Here's the drawing with two shaded views (mm, measured from the low corner). I have some questions. Give positions to 0.01 mm unless a question says otherwise; leave off trailing zeros. Write each loop counter-clockwise with the first axis right and the second up, starting at its lowest first coordinate (ties: lowest second). Pieces come first, ordered by that corner, then holes. Notation, with made-up numbers: (31.25, -9) - (38.25, -9) arc R4 cw to (38.25, -3) - close; hole circle Ø2 at (24.5, 18). An arc over 180 degrees is marked (long way). Write item = value, one per line.
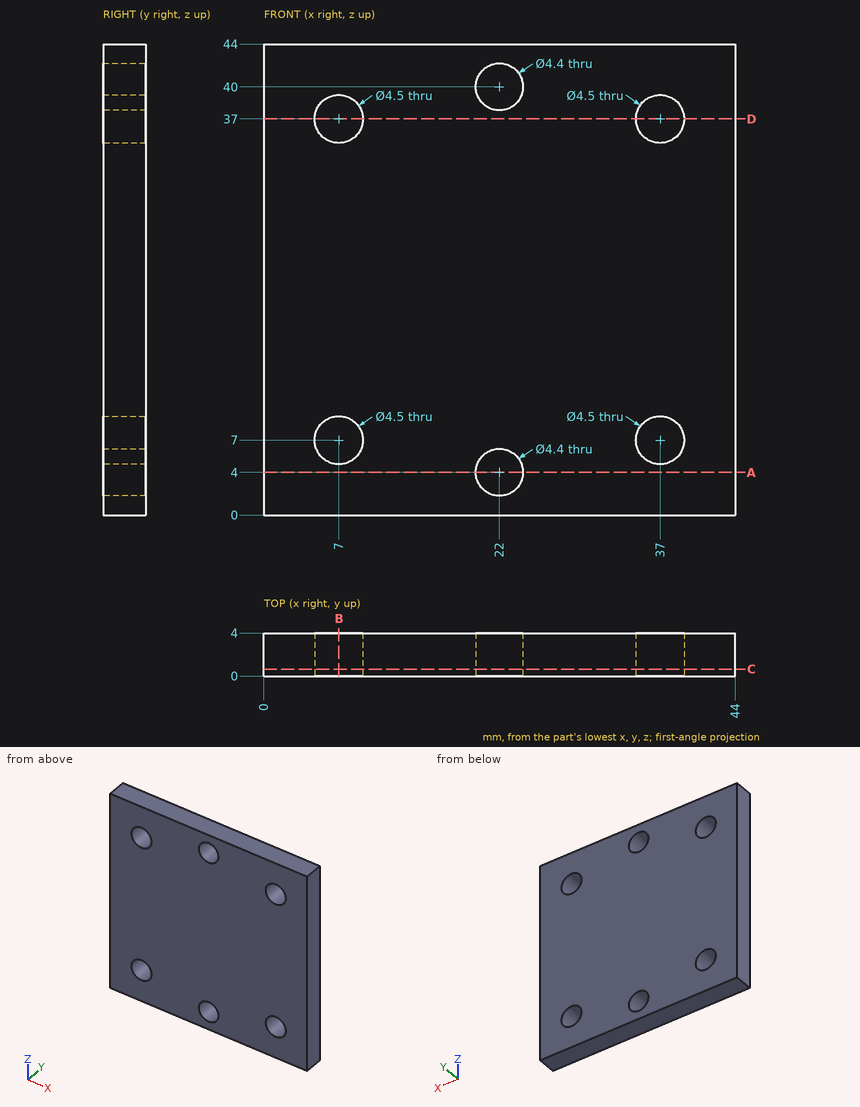
1. For pin 1 (3 mm diameter, centred on x = 25.5, z = 36.5, fed in from -Y); pin 2 (3.5 mm diameter, centred on x = 37, z = 37, fed in from -Y), each with a flat end and sliding along its axis, tell me the tip position at first contact or that it passes through.
Filled sheet:
pin_1 = 0
pin_2 = through
2. If we section it at C-C, the plane y = 0.65: Please give me the cut outline in (x, z), and give its area (3 significant figures).
Filled sheet:
outline = (0, 0) - (44, 0) - (44, 44) - (0, 44) - close; hole circle Ø4.5 at (7, 7); hole circle Ø4.5 at (7, 37); hole circle Ø4.4 at (22, 4); hole circle Ø4.4 at (22, 40); hole circle Ø4.5 at (37, 7); hole circle Ø4.5 at (37, 37)
area = 1,840 mm2
3. If we section it at A-A, the plane z = 4: Please give me the cut outline in (x, y).
Filled sheet:
outline = (0, 0) - (19.8, 0) - (19.8, 4) - (0, 4) - close; (24.2, 0) - (44, 0) - (44, 4) - (24.2, 4) - close
4. If we section it at B-B, the plane x = 7: Please give me the cut outline in (y, z).
Filled sheet:
outline = (0, 0) - (4, 0) - (4, 4.75) - (0, 4.75) - close; (0, 9.25) - (4, 9.25) - (4, 34.75) - (0, 34.75) - close; (0, 39.25) - (4, 39.25) - (4, 44) - (0, 44) - close
5. If we section it at D-D, the plane z = 37: Please give me the cut outline in (x, y).
Filled sheet:
outline = (0, 0) - (4.75, 0) - (4.75, 4) - (0, 4) - close; (9.25, 0) - (34.75, 0) - (34.75, 4) - (9.25, 4) - close; (39.25, 0) - (44, 0) - (44, 4) - (39.25, 4) - close
6. I need wall thicknesses on line 1 (X direction, y = 1.8, z = 37); line 2 (X direction, y = 1.15, z = 8); line 3 (X direction, y = 2.35, z = 4). Which ranges of each line are inside material? Lowest first, please.
Filled sheet:
line_1 = 0 to 4.75, 9.25 to 34.75, 39.25 to 44
line_2 = 0 to 4.98, 9.02 to 34.98, 39.02 to 44
line_3 = 0 to 19.8, 24.2 to 44
